from build123d import *

# Parameters (mm, degrees)
SKETCH1_W                        = 140
SKETCH1_H                        = 115
BOSS_EXTRUDE1_DEPTH              = 80
SKETCH2_W                        = 126
SKETCH2_H                        = 101
CUT_EXTRUDE1_DEPTH               = 70
M10X1_0_TAPPED_HOLE1_D           = 9
M10X1_0_TAPPED_HOLE1_DEPTH       = 23
M10X1_0_TAPPED_HOLE1_CBORE_D     = 10
M10X1_0_TAPPED_HOLE1_CBORE_DEPTH = 20
M10X1_0_TAPPED_HOLE1_TIP         = 2.703872786
M10X1_0_TAPPED_HOLE2_D           = 9
M10X1_0_TAPPED_HOLE2_DEPTH       = 23
M10X1_0_TAPPED_HOLE2_CBORE_D     = 10
M10X1_0_TAPPED_HOLE2_CBORE_DEPTH = 20
M10X1_0_TAPPED_HOLE2_TIP         = 2.703872786


with BuildPart() as part:
    # Sketch1 → Boss-Extrude1 (new body)
    with BuildSketch(Plane(origin=(0, 0, 0), x_dir=(1, 0, 0), z_dir=(0, 1, 0))):
        with Locations((-2.716319444, -3.909068683)):
            Rectangle(SKETCH1_W, SKETCH1_H)
    extrude(amount=BOSS_EXTRUDE1_DEPTH)

    # Sketch2 → Cut-Extrude1 (cut)
    with BuildSketch(Plane(origin=(0, 80, 0), x_dir=(1, 0, 0), z_dir=(0, 1, 0))):
        with Locations((-2.716319444, -3.909068683)):
            Rectangle(SKETCH2_W, SKETCH2_H)
    extrude(amount=-CUT_EXTRUDE1_DEPTH, mode=Mode.SUBTRACT)

    # M10x1.0 Tapped Hole1
    with Locations(Plane(origin=(-17.716319444, 50, -53.590931317), x_dir=(-1, 0, 0), z_dir=(0, 0, -1))):
        with Locations((0, 0), (-60, 0)):
            CounterBoreHole(M10X1_0_TAPPED_HOLE1_D / 2, M10X1_0_TAPPED_HOLE1_CBORE_D / 2, M10X1_0_TAPPED_HOLE1_CBORE_DEPTH, depth=M10X1_0_TAPPED_HOLE1_DEPTH)
            with Locations((0, 0, -(M10X1_0_TAPPED_HOLE1_DEPTH + M10X1_0_TAPPED_HOLE1_TIP / 2))):  # 118° drill point
                Cone(0, M10X1_0_TAPPED_HOLE1_D / 2, M10X1_0_TAPPED_HOLE1_TIP, mode=Mode.SUBTRACT)

    # M10x1.0 Tapped Hole2
    with Locations(Plane(origin=(67.283680556, 40, 11.409068683), x_dir=(0, 0, 1), z_dir=(1, 0, 0))):
        with Locations((0, 0)):
            CounterBoreHole(M10X1_0_TAPPED_HOLE2_D / 2, M10X1_0_TAPPED_HOLE2_CBORE_D / 2, M10X1_0_TAPPED_HOLE2_CBORE_DEPTH, depth=M10X1_0_TAPPED_HOLE2_DEPTH)
            with Locations((0, 0, -(M10X1_0_TAPPED_HOLE2_DEPTH + M10X1_0_TAPPED_HOLE2_TIP / 2))):  # 118° drill point
                Cone(0, M10X1_0_TAPPED_HOLE2_D / 2, M10X1_0_TAPPED_HOLE2_TIP, mode=Mode.SUBTRACT)


solid = part.part
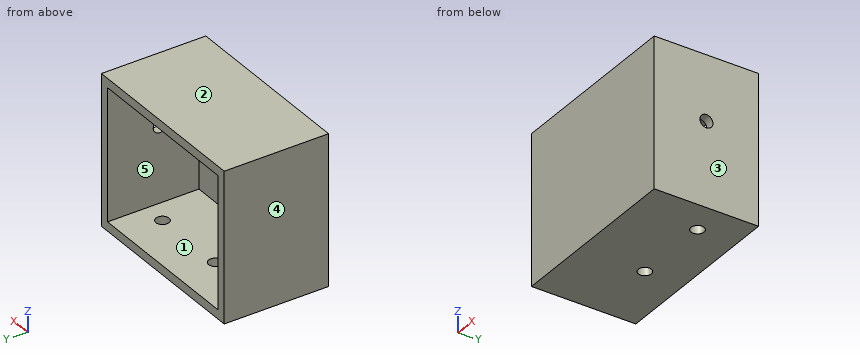
Here's how the part is built. I have some questions about the finished solid (model axes, mm). Face numbers are marked on the shaded views. A direction names the side the tool comes from. Give positions to 0.01 mm unless a question says otherwise; leave off trailing zeros. Loops run counter-clockwise (first coordinate to the right, second up) from the corner with the lowest first, then second, coordinate; pieces in that order, holes last. Notation, with made-up numbers: (70, 36) -> (120, 36) arc R18 ccw to (120, 43) -> close; hole circle Ø11 at (39, 64.25). An arc over 180 degrees is marked (long way). One line per item, written item: value.
Q1. If I drill on line 1 along Z through (x, y) = (-8.5, 36); line 2 along X through (y, z) = (64.5, 33.5); line 3 along Z through (x, y) = (65, 40), over which ranges is the centre line in solid material (lowest first)?
Answers follow:
line 1: -53.59 to -46.59, 54.41 to 61.41
line 2: -72.72 to -65.72, 60.28 to 67.28
line 3: -53.59 to 6.41, 16.41 to 61.41
Q2. On a 3-axis mill with a long thin cutter (end or side, diameter ignored), from which of +Z, -Z, +X, -X, +Y, -Y can I reach the whole of each face in a straight line? I mean the marked faces 4 and 5. Say none if no direction works.
Answers follow:
face 4: +Z, -Z, -X, +Y, -Y
face 5: +Y
Q3. Suppose I cut it at A-A on y = 50. Please give me the cut outline in (x, z).
Answers follow:
outline: (-72.72, -53.59) -> (-22.72, -53.59) -> (-22.72, -46.59) -> (-65.72, -46.59) -> (-65.72, 54.41) -> (60.28, 54.41) -> (60.28, -46.59) -> (47.28, -46.59) -> (47.28, -53.59) -> (67.28, -53.59) -> (67.28, 61.41) -> (-72.72, 61.41) -> close; (-12.72, -53.59) -> (37.28, -53.59) -> (37.28, -46.59) -> (-12.72, -46.59) -> close
Q4. Suppose I cut it at B-B on y = 74.5. Please give me the cut outline in (x, z).
Answers follow:
outline: (-72.72, -53.59) -> (67.28, -53.59) -> (67.28, 61.41) -> (-72.72, 61.41) -> close; hole (-65.72, -46.59) -> (60.28, -46.59) -> (60.28, 54.41) -> (-65.72, 54.41) -> close
Q5. Suppose I cut it at C-C on z = 26.5. Please give me the cut outline in (x, y), then the cut area to 3 significant figures.
Answers follow:
outline: (-72.72, 0) -> (67.28, 0) -> (67.28, 80) -> (60.28, 80) -> (60.28, 10) -> (-65.72, 10) -> (-65.72, 80) -> (-72.72, 80) -> close
area: 2,380 mm^2
Q6. Suppose I cut it at D-D on y = 40. Please give me the cut outline in (x, z).
Answers follow:
outline: (-72.72, -53.59) -> (67.28, -53.59) -> (67.28, 6.41) -> (60.28, 6.41) -> (60.28, -46.59) -> (-65.72, -46.59) -> (-65.72, 54.41) -> (60.28, 54.41) -> (60.28, 16.41) -> (67.28, 16.41) -> (67.28, 61.41) -> (-72.72, 61.41) -> close
Q7. I'm going to push flat-ended pins straight in: pin 1 Ø9 at (x, y) = (42.28, 50) entering from -Z; pin 2 Ø8 at (x, z) = (24.5, 2.5) entering from +Y; pin 3 Ø6 at (y, z) = (40, 11.41) entering from +X. Where does each tip first touch, or does it pass through?
Answers follow:
pin 1: z = 54.41
pin 2: y = 10
pin 3: x = -65.72
Q8. We'd pull the mould along X, two halves only. Please class the marked faces 1, 2 and 3: pulls with the +X half, pulls with the -X half, needs draft (parallel to the pull), parting line crosses it, or undercut.
Answers follow:
face 1: undercut
face 2: needs draft
face 3: pulls with the +X half
